Input: part model. Units: mm. Frame: model coordinates. A direction names the side the tool comes from. Give positions to 0.01 mm unless a question says otherwise; leave off trailing zeros. Loops run counter-clockwise (first coordinate to the right, second up) from the corner with the lowest first, then second, coordinate; pieces in that order, holes last. Notation, with made-up numbers: M -32.5,56.25 L 15.5,56.25 A8 cw 15.5,67.25 Z; hole C 60.5,-35 d11. An arc over 180 degrees is marked long. Use CSV: the item, a comma, the result in double quotes. Start each with the question number.
from build123d import *

# Parameters (mm, degrees)
SKETCH_W          = 36
SKETCH_H          = 21
SKETCH_R          = 2
PAD_DEPTH         = 24
SKETCH001_W       = 6.5
SKETCH001_H       = 18
POCKET_DEPTH      = 21
POCKET001_DEPTH   = 24
SKETCH003_W       = 6
SKETCH003_H       = 6
SKETCH003_R       = 2
PAD001_DEPTH      = 1.5
PAD001_DEPTH_BACK = 22.5


with BuildPart() as part:
    # Sketch → Pad (new body)
    with BuildSketch(Plane.XY):
        with Locations((18, 10.5)):
            Rectangle(SKETCH_W, SKETCH_H)
        with Locations((3, 16.5)):
            Circle(SKETCH_R, mode=Mode.SUBTRACT)
        with Locations((3, 10.5)):
            Circle(SKETCH_R, mode=Mode.SUBTRACT)
        with Locations((3, 4.5)):
            Circle(SKETCH_R, mode=Mode.SUBTRACT)
        with Locations((26, 10.5)):
            Circle(SKETCH_R, mode=Mode.SUBTRACT)
    extrude(amount=PAD_DEPTH)

    # Sketch001 → Pocket (cut)
    with BuildSketch(Plane.XZ):
        with Locations((3.25, 12)):
            Rectangle(SKETCH001_W, SKETCH001_H)
    extrude(amount=-POCKET_DEPTH, mode=Mode.SUBTRACT)

    # Sketch002 → Pocket001 (cut)
    with BuildSketch(Plane(origin=(0, 0, 0), x_dir=(1, 0, 0), z_dir=(0, 0, -1))):
        Polygon((0, -18.1), (2.9, -21), (0, -21), align=None)
        Polygon((33.1, -21), (36, -18.1), (36, -21), align=None)
        Polygon((36, -2.9), (33.1, 0), (36, 0), align=None)
        Polygon((2.9, 0), (0, -2.9), (0, 0), align=None)
    extrude(amount=-POCKET001_DEPTH, mode=Mode.SUBTRACT)

    # Sketch003 → Pad001 (new body, two sides)
    with BuildSketch(Plane.XZ) as pad001_sk:
        with Locations((9.5, 18)):
            Rectangle(SKETCH003_W, SKETCH003_H)
        with Locations((9.5, 18)):
            Circle(SKETCH003_R, mode=Mode.SUBTRACT)
        with Locations((9.5, 6)):
            Rectangle(SKETCH003_W, SKETCH003_H)
        with Locations((9.5, 6)):
            Circle(SKETCH003_R, mode=Mode.SUBTRACT)
        with Locations((27.5, 18)):
            Rectangle(SKETCH003_W, SKETCH003_H)
        with Locations((27.5, 18)):
            Circle(SKETCH003_R, mode=Mode.SUBTRACT)
        with Locations((27.5, 6)):
            Rectangle(SKETCH003_W, SKETCH003_H)
        with Locations((27.5, 6)):
            Circle(SKETCH003_R, mode=Mode.SUBTRACT)
    extrude(amount=PAD001_DEPTH)
    extrude(pad001_sk.sketch, amount=-PAD001_DEPTH_BACK)


solid = part.part
Item 1: Section C-C (y = 10.5). State how many separate pieces and enclosed holes the cut face has, then the cut area to 3 significant figures.
Item 2: Mould query, pull axis Y, two halves, no side actions, for faces 4 (the flat face through (26, 10, 15)), 5 (the flat face through (25, 22.5, 6)), 6 (the flat face through (27, -1, 3)). Classes: +Y half, -Y half, draft (parallel to the pull), parting line (faces both ways), or undercut.
Item 3: Section A-A (y = 4.5). Output: boundary loops of the cut face in (x, z).
Item 4: Set-up query: faces 1 (the flat face through (24.5, 22, 18)), 2 (the cylindrical face through (9.24, 21.74, 19.983)), 3 (the cylindrical face through (24.002, 10.588, 11.832)). Return all of +Z, -Z, +X, -X, +Y, -Y with unobstructed straight access to the full face (end or side cutting, diameter ignored); none if empty.
Item 5: Section B-B (z = 13.5). Output: boundary loops of the cut face in (x, y), then the cut area to 3 significant figures.
Item 6: First-contact query: pin 1 Ø1.3 at (y, z) = (10, 19.5) entering from -X; pin 2 Ø5 at (x, z) = (21, 5) entering from +Y; pin 3 Ø0.8 at (x, y) = (28.5, -0.5) entering from -Z. Flat tips, straight axial feed; report the tip coordinate or a pass-through.
Item 7: Section D-D (y = 13.25). Output: boundary loops of the cut face in (x, z), then the cut area to 3 significant figures.
Item 8: Material intervals for line 1 (Z direction, x = 27.5, y = 22); line 2 (Y direction, x = 3, z = 23.1); line 3 (X direction, y = 10.6, z = 6), sorted ascending.
Recorded:
1,separate pieces,"4"
1,enclosed holes,"2"
1,area,"652 mm²"
2,face 4,"undercut"
2,face 5,"+Y half"
2,face 6,"draft"
3,outline,"M 0,0 L 1,0 L 1,3 L 0,3 Z; M 0,21 L 1,21 L 1,24 L 0,24 Z; M 5,0 L 36,0 L 36,24 L 5,24 L 5,21 L 6.5,21 L 6.5,3 L 5,3 Z"
4,face 1,"+Z, -Z, +Y"
4,face 2,"+Y"
4,face 3,"none"
5,outline,"M 6.5,0 L 33.1,0 L 36,2.9 L 36,18.1 L 33.1,21 L 6.5,21 Z; hole C 26,10.5 d4"
5,area,"599 mm²"
6,pin 1,"x = 6.5"
6,pin 2,"y = 21"
6,pin 3,"z = 3"
7,outline,"M 0,0 L 36,0 L 36,24 L 0,24 L 0,21 L 6.5,21 L 6.5,3 L 0,3 Z"
7,area,"747 mm²"
8,line 1,"3 to 4, 8 to 9, 15 to 16, 20 to 21"
8,line 2,"0 to 2.5, 6.5 to 8.5, 12.5 to 14.5, 18.5 to 21"
8,line 3,"6.5 to 24, 24.5 to 25.5, 28 to 36"
